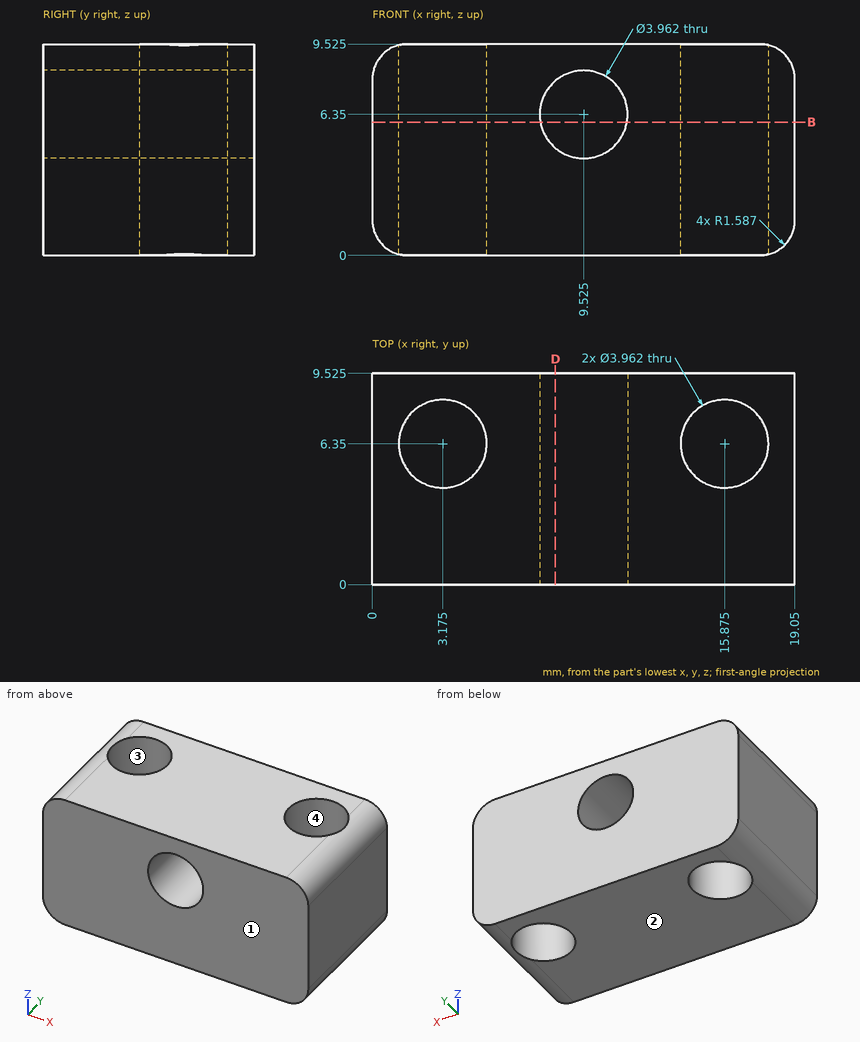
Check sheet for the drawn part. Datum: minimum x, y, z corner. Units: mm. Round coordinates to 2 decimals unless told otherwise and drop trailing zeros. Loops run counter-clockwise (first coordinate to the right, second up) from the corner with the lowest first, then second, coordinate; pieces in that order, holes last. Notation, with made-up numbers: (-30.75, 8) -> (-14.75, 8) arc R23 ccw to (-14.75, 47) -> close; hole circle Ø5 at (-29, 71). An arc over 180 degrees is marked (long way). Put each result on its own line as item: value. Start each with the question number.
1. Section check D-D (x = 8.25). Enter the section's corners in (y, z) (1 decimal).
2. Draft check along Y on the marked faces 1, 2, 3 and 4. Enter one of: +Y half, -Y half, draft (parallel to the pull), parting line (faces both ways), or undercut.
3. Section check B-B (z = 6). Give the number of separate pieces and of enclosed holes in the cut face, plus the area to 3 significant figures.
4. Scan lines: probe 1 along X at (y, z) = (6.35, 2.75); probe 2 along X at (y, z) = (2.5, 6.35); probe 3 along X at (y, z) = (6, 1.5) (1 decimal). Record each from-to range of solid material in increasing order.
Findings:
1. outline: (0, 0) -> (9.5, 0) -> (9.5, 4.8) -> (0, 4.8) -> close; (0, 7.9) -> (9.5, 7.9) -> (9.5, 9.5) -> (0, 9.5) -> close
2. face 1: -Y half
2. face 2: draft
2. face 3: undercut
2. face 4: undercut
3. separate pieces: 2
3. enclosed holes: 2
3. area: 120 mm^2
4. probe 1: x = 0 to 1.19, 5.16 to 13.89, 17.86 to 19.05
4. probe 2: x = 0 to 7.54, 11.51 to 19.05
4. probe 3: x = 0 to 1.2, 5.1 to 13.9, 17.8 to 19
